Here's how the part is built. I have some questions about the finished solid (model axes, mm). Coordinates: 2 decimals unless noted, no trailing zeros. Order: outer loops, then holes, each group sorted by start corner. A loop starts at its lowest first (then second) coordinate and runs counter-clockwise, first axis right, second up. Notation, with made-up numbers: (20.5, 31.25) - (40.5, 31.25) arc R25 cw to (40.5, 57.25) - close; hole circle Ø5 at (36.25, 6). An arc over 180 degrees is marked (long way). Answer in a Markdown table with one row per item. Add a question column.
Item 1: Will these pins go through, and if not, where does the flat tip stop? pin 1 Ø3 at (x, y) = (2.8, 2.8) entering from +Z; pin 2 Ø8 at (x, y) = (12.5, 4.5) entering from -Z.
Item 2: I want a section at A-A (x = 2.8). Please give me the cut outline in (y, z), plus the area to 3 significant figures.
Item 3: I want a section at C-C (z = 2.5). Please give me the cut outline in (x, y).
Item 4: If I drill on line 1 along X through (y, z) = (13.1, 4.75); line 2 along X through (y, z) = (2.8, 4.75); line 3 along Y through (x, z) = (25, 5.25), over which ranges is the centre line in solid material (lowest first)? Write a range as from..to.
Item 5: I want a section at B-B (y = 2.8). Please give me the cut outline in (x, z).
Item 6: Thinking about a two-plate mould opening in X: for faces 1 (the flat face through (14, 8, 0)), 2 (the cylindrical face through (25.336, 14.613, 5.078)), 3 (the flat face through (27.8, 8, 5)), which applies, +X half, -X half, draft (parallel to the pull), parting line (faces both ways), or undercut?
```python
from build123d import *

# Parameters (mm, degrees)
SKETCH_2_W      = 27.8
SKETCH_2_H      = 15.9
SKETCH_2_R      = 1.55
EXTRUDE_1_DEPTH = 10.3


with BuildPart() as part:
    # ｽｹｯﾁ2 → ﾎﾞｽ - 押し出し1 (new body)
    with BuildSketch(Plane.XY):
        with Locations((13.9, 7.95)):
            Rectangle(SKETCH_2_W, SKETCH_2_H)
        with Locations(Location((2.8, 2.8, 0), (0, 0, 180))):
            Circle(SKETCH_2_R, mode=Mode.SUBTRACT)
        with Locations(Location((25, 13.1, 0), (0, 0, 180))):
            Circle(SKETCH_2_R, mode=Mode.SUBTRACT)
    extrude(amount=EXTRUDE_1_DEPTH)


solid = part.part
```
Values follow:
| question | item | result |
|---|---|---|
| 1 | pin 1 | passes through |
| 1 | pin 2 | stops at z = 0 |
| 2 | outline | (0, 0) - (1.25, 0) - (1.25, 10.3) - (0, 10.3) - close; (4.35, 0) - (15.9, 0) - (15.9, 10.3) - (4.35, 10.3) - close |
| 2 | area | 132 mm^2 |
| 3 | outline | (0, 0) - (27.8, 0) - (27.8, 15.9) - (0, 15.9) - close; hole circle Ø3.1 at (2.8, 2.8); hole circle Ø3.1 at (25, 13.1) |
| 4 | line 1 | x = 0..23.45, 26.55..27.8 |
| 4 | line 2 | x = 0..1.25, 4.35..27.8 |
| 4 | line 3 | y = 0..11.55, 14.65..15.9 |
| 5 | outline | (0, 0) - (1.25, 0) - (1.25, 10.3) - (0, 10.3) - close; (4.35, 0) - (27.8, 0) - (27.8, 10.3) - (4.35, 10.3) - close |
| 6 | face 1 | draft |
| 6 | face 2 | undercut |
| 6 | face 3 | +X half |
